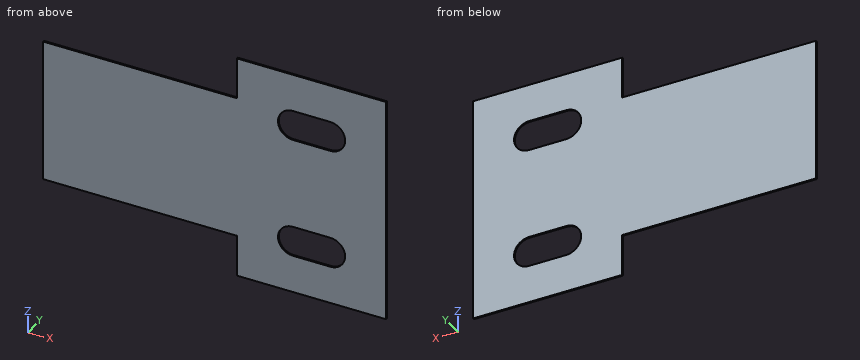
from build123d import *

# Parameters (mm, degrees)
BOSS_EXTRUDE1_DEPTH = 0.05


with BuildPart() as part:
    # Sketch1 → Boss-Extrude1 (new, symmetric)
    with BuildSketch(Plane(origin=(0, 0, 0), x_dir=(1, 0, 0), z_dir=(0, 1, 0))):
        Polygon((-6.778814753, -5.787261175), (6.221185247, -5.787261175), (6.221185247, -8.537261175), (16.221185247, -8.537261175), (16.221185247, 6.462738825), (6.221185247, 6.462738825), (6.221185247, 3.712738825), (-6.778814753, 3.712738825), align=None)
        with BuildLine():
            Line((12.471185247, 3.962738825), (9.971185247, 3.962738825))
            ThreePointArc((9.971185247, 3.962738825), (8.971185247, 2.962738825), (9.971185247, 1.962738825))
            Line((9.971185247, 1.962738825), (12.471185247, 1.962738825))
            ThreePointArc((12.471185247, 1.962738825), (13.471185247, 2.962738825), (12.471185247, 3.962738825))
        make_face(mode=Mode.SUBTRACT)
        with BuildLine():
            Line((12.471185247, -4.037261175), (9.971185247, -4.037261175))
            ThreePointArc((9.971185247, -4.037261175), (8.971185247, -5.037261175), (9.971185247, -6.037261175))
            Line((9.971185247, -6.037261175), (12.471185247, -6.037261175))
            ThreePointArc((12.471185247, -6.037261175), (13.471185247, -5.037261175), (12.471185247, -4.037261175))
        make_face(mode=Mode.SUBTRACT)
    extrude(amount=BOSS_EXTRUDE1_DEPTH, both=True)


solid = part.part
Can you work these out from the model? Positions are in its coordinate system, mm. Coordinates: 2 decimals unless noted, no trailing zeros. Order: outer loops, then holes, each group sorted by start corner. A loop starts at its lowest first (then second) coordinate and runs counter-clockwise, first axis right, second up. Notation, with made-up numbers: (-35.75, -23) -> (-12.75, -23) arc R19 ccw to (-12.75, -19) -> close; hole circle Ø8 at (-14.5, 38.5). An arc over 180 degrees is marked (long way). Use one line per item in the form item = value.
Q1. I need wall thicknesses on L1, parallel to X at y = 0, z = -5; L2, parallel to Z at x = -2.5, y = 0; L3, parallel to X at y = 0, z = -3.75. Which ranges of each line are inside material? Lowest first, please.
From the geometry:
L1 = 6.22 to 16.22
L2 = -3.71 to 5.79
L3 = 6.22 to 9.35, 13.09 to 16.22
Q2. Imagine slicing it at D-D, the plane z = 7.5. List the corners of the cut face in (x, y) for me.
From the geometry:
outline = (6.22, -0.05) -> (16.22, -0.05) -> (16.22, 0.05) -> (6.22, 0.05) -> close
Q3. Imagine slicing it at C-C, the plane z = 5. List the corners of the cut face in (x, y) for me.
From the geometry:
outline = (-6.78, -0.05) -> (8.97, -0.05) -> (8.97, 0.05) -> (-6.78, 0.05) -> close; (13.47, -0.05) -> (16.22, -0.05) -> (16.22, 0.05) -> (13.47, 0.05) -> close
Q4. Imagine slicing it at B-B, the plane y = 0. List the corners of the cut face in (x, z) for me.
From the geometry:
outline = (-6.78, -3.71) -> (6.22, -3.71) -> (6.22, -6.46) -> (16.22, -6.46) -> (16.22, 8.54) -> (6.22, 8.54) -> (6.22, 5.79) -> (-6.78, 5.79) -> close; hole (9.97, -3.96) -> (12.47, -3.96) arc R1 ccw to (12.47, -1.96) -> (9.97, -1.96) arc R1 ccw to start; hole (9.97, 4.04) -> (12.47, 4.04) arc R1 ccw to (12.47, 6.04) -> (9.97, 6.04) arc R1 ccw to start
Q5. Imagine slicing it at A-A, the plane x = 10.5. List the corners of the cut face in (y, z) for me, then the cut area to 3 significant figures.
From the geometry:
outline = (-0.05, -6.46) -> (0.05, -6.46) -> (0.05, -3.96) -> (-0.05, -3.96) -> close; (-0.05, -1.96) -> (0.05, -1.96) -> (0.05, 4.04) -> (-0.05, 4.04) -> close; (-0.05, 6.04) -> (0.05, 6.04) -> (0.05, 8.54) -> (-0.05, 8.54) -> close
area = 1.10 mm²
